Autodesk Inventor part; units mm, degrees
ref_plane "YZ Plane" through (0, 0, 0) normal (1, 0, 0) x (0, 1, 0)
ref_plane "XZ Plane" through (0, 0, 0) normal (0, 1, 0) x (-1, 0, 0)
ref_plane "XY Plane" through (0, 0, 0) normal (0, 0, 1) x (1, 0, 0)
sketch "Sketch1" plane through (0, 0, 0) normal (0, 0, 1) x (1, 0, 0)
  line L0 (-4.5, -12.5) -> (4.5, -12.5)
  line L1 (4.5, -12.5) -> (4.5, 12.5)
  line L2 (4.5, 12.5) -> (-4.5, 12.5)
  line L3 (-4.5, 12.5) -> (-4.5, -12.5)
  line L4 (-4.5, -12.5) -> (4.5, 12.5) construction
  line L5 (4.5, -12.5) -> (-4.5, 12.5) construction
  point P0 (0, 0)
  dimension "d0" = 9
  dimension "d1" = 25
extrude "Extrusion1" add sketch "Sketch1" along normal blind 2
sketch "Sketch2" plane through (-4.5, -12.5, 0) normal (0, -1, 0) x (1, 0, 0)
  line L0 (4.5, 0) -> (4.5, 2) construction
  line L1 (9, 2) -> (0, 2) construction
  line L2 (0, 0) -> (0, 2) construction
  line L3 (0, 1) -> (9, 1) construction
  line L4 (2.4, 0.25) -> (6.6, 0.25)
  line L5 (6.6, 0.25) -> (6.6, 1.75)
  line L6 (6.6, 1.75) -> (2.4, 1.75)
  line L7 (2.4, 1.75) -> (2.4, 0.25)
  line L8 (2.4, 0.25) -> (6.6, 1.75) construction
  line L9 (6.6, 0.25) -> (2.4, 1.75) construction
  point P0 (4.5, 1)
  dimension "d4" = 4.2
  dimension "d5" = 1.5
extrude "Extrusion2" cut sketch "Sketch2" against normal blind 254
fillet "Fillet1" radius 0.3 4 edges at (-2.1, 0, 0.25) (2.1, 0, 0.25) (-2.1, 0, 1.75) (2.1, 0, 1.75)
fillet "Fillet2" radius 0.3 12 edges at (4.5, 0, 0) (4.5, -12.5, 1) (4.5, 0, 2) (0, -12.5, 0) (0, -12.5, 2) (4.5, 12.5, 1) (0, 12.5, 0) (0, 12.5, 2) (-4.5, 12.5, 1) (-4.5, 0, 0) (-4.5, 0, 2) (-4.5, -12.5, 1)
properties part number "OTOSGuard"
Check sheet for the modelled part. Datum: model origin and axes. Units: mm. A direction names the side the tool comes from. Coordinates: 2 decimals unless noted, no trailing zeros. Order: outer loops, then holes, each group sorted by start corner. A loop starts at its lowest first (then second) coordinate and runs counter-clockwise, first axis right, second up. Notation, with made-up numbers: (32.25, 57.25) -> (63.25, 57.25) arc R21 ccw to (63.25, 95.25) -> close; hole circle Ø7 at (0, 35). An arc over 180 degrees is marked (long way). Write each question's results on one line, items separated by ' | '. Start each with the question number.
1) Material ranges on line 1 along X through (y, z) = (7, 0.6); line 2 along Z through (x, y) = (-0.5, 1.5); line 3 along Z through (x, y) = (4.25, -8), recorded low to high.
2) Draft check along X on faces 3 (the face through (0, 0, 2)), 4 (the face through (4.5, 0, 1)), 5 (the face through (0, 0, 0.25)). Enter one of: pulls with the +X half, pulls with the -X half, needs draft (parallel to the pull), parting line crosses it, or undercut.
3) Set-up check for faces 1 (the face through (-2.1, 0, 1)), 2 (the face through (-3, -12.5, 1)): record each of +Z, -Z, +X, -X, +Y, -Y from which the full face is reachable in a straight line by a thin tool's end or side.
4) Section check A-A (z = 0.9). Enter the section's corners in (x, y), and give its area (3 significant figures).
5) Depth check by flat-ended pin: pin 1 (1.1 mm diameter, centred on x = 0, y = -6, fed in from -Z). Enter the tip coordinate at first touch or a pass-through.
6) Section check B-B (y = 6.75). Enter the section's corners in (x, z), and give its area (3 significant figures).
Checked values:
1) line 1: -4.5 to -2.1, 2.1 to 4.5 | line 2: 0 to 0.25, 1.75 to 2 | line 3: 0 to 2
2) face 3: needs draft | face 4: pulls with the +X half | face 5: undercut
3) face 1: +Y, -Y | face 2: +Z, -Z, +X, -X, -Y
4) outline: (-4.5, -12.2) arc R0.3 ccw to (-4.2, -12.5) -> (-2.1, -12.5) -> (-2.1, 12.5) -> (-4.2, 12.5) arc R0.3 ccw to (-4.5, 12.2) -> close; (2.1, -12.5) -> (4.2, -12.5) arc R0.3 ccw to (4.5, -12.2) -> (4.5, 12.2) arc R0.3 ccw to (4.2, 12.5) -> (2.1, 12.5) -> close | area: 120 mm²
5) pin 1: z = 0
6) outline: (-4.5, 0.3) arc R0.3 ccw to (-4.2, 0) -> (4.2, 0) arc R0.3 ccw to (4.5, 0.3) -> (4.5, 1.7) arc R0.3 ccw to (4.2, 2) -> (-4.2, 2) arc R0.3 ccw to (-4.5, 1.7) -> close; hole (-2.1, 0.55) arc R0.3 ccw to (-1.8, 0.25) -> (1.8, 0.25) arc R0.3 ccw to (2.1, 0.55) -> (2.1, 1.45) arc R0.3 ccw to (1.8, 1.75) -> (-1.8, 1.75) arc R0.3 ccw to (-2.1, 1.45) -> close | area: 11.7 mm²
